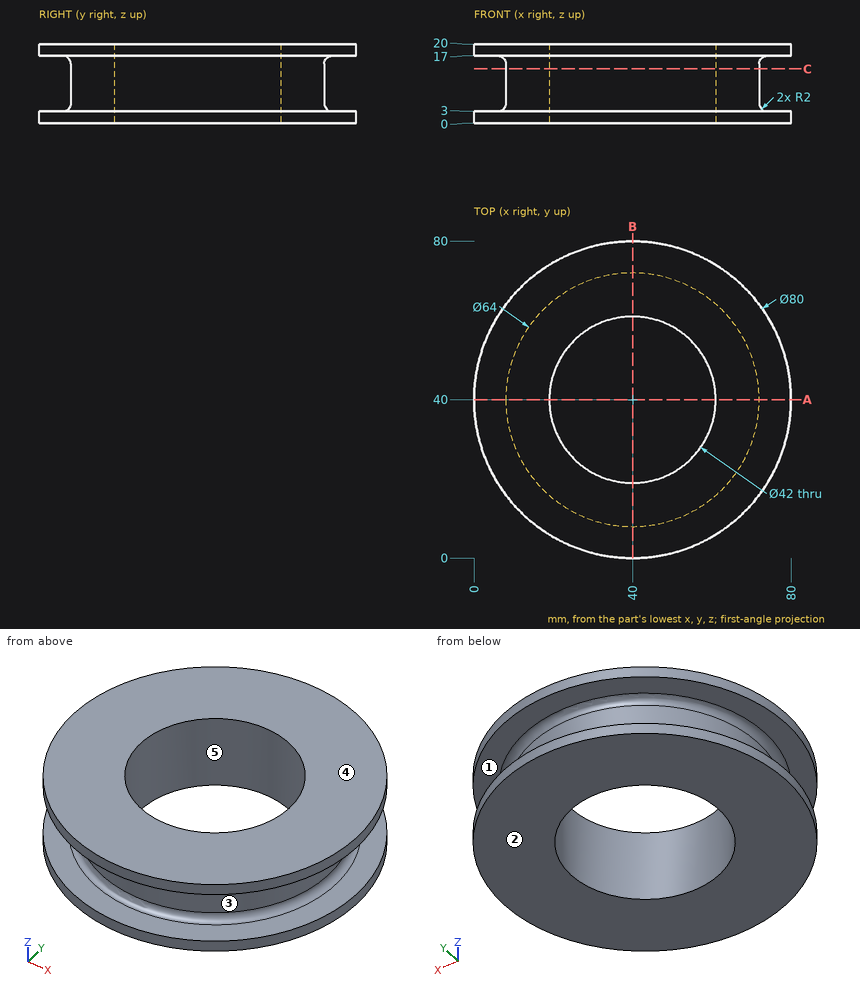
Study the drawing (mm; zero at the part's minimum x, y, z) and answer. A direction names the side the tool comes from. Give positions to 0.01 mm unless a question says otherwise; leave off trailing zeros. Loops run counter-clockwise (first coordinate to the right, second up) from the corner with the lowest first, then second, coordinate; pieces in that order, holes last. Notation, with made-up numbers: (76.5, 56) - (80.5, 56) arc R36 cw to (80.5, 92) - close; hole circle Ø10 at (-1, 61.25). An arc over 180 degrees is marked (long way). Answer in a Markdown table with one row per item. Add a question column.
Q1. Each of these flat-tipped pins is pushed along its axis until it touches: P1, Ø2, axis at y = 15.5, z = 2.5, coming from the +X side; P2, Ø5, axis at x = 24, z = 9.5, coming from the +Y side; P3, Ø1.5, axis at x = 35.5, y = 20.5, coming from the -Z side; P4, Ø3, axis at x = 19.5, z = 11, coming from the +Y side. Where does it stop, or does it pass through?
Q2. The part is cut by section C-C (z = 13.75). Determine the outline of the cut face in (x, y), and give its area (3 significant figures).
Q3. A tool of negligible diameter and unlimited length cuts with its end or side. For the marked faces 1 and 2, from which of +Z, -Z, +X, -X, +Y, -Y can it reach the whole face along a straight path? Write none if from no direction.
Q4. Consider line 1 along Y through (x, z) = (40, 10.75); line 2 along Y through (x, z) = (40, 4.5); line 3 along X through (y, z) = (21, 6.5). Determine where each line is inside the solid, lowest interval first.
Q5. Determine the mould class of the marked faces 3, 4 and 5 for opening direction X: released by +X, released by -X, zero draft, split by the parting line, or undercut.
Q6. The part is cut by section A-A (y = 40). Determine the outline of the cut face in (x, z), and give its area (3 significant figures).
Solution:
| question | item | result |
|---|---|---|
| 1 | P1 | stops at x = 72.37 |
| 1 | P2 | stops at y = 69.01 |
| 1 | P3 | passes through |
| 1 | P4 | stops at y = 65.75 |
| 2 | outline | circle Ø64 at (40, 40); hole circle Ø42 at (40, 40) |
| 2 | area | 1,830 mm² |
| 3 | face 1 | none |
| 3 | face 2 | -Z, +X, -X, +Y, -Y |
| 4 | line 1 | y = 8 to 19, 61 to 72 |
| 4 | line 2 | y = 7.94 to 19, 61 to 72.06 |
| 4 | line 3 | x = 14.25 to 31.06, 48.94 to 65.75 |
| 5 | face 3 | split by the parting line |
| 5 | face 4 | zero draft |
| 5 | face 5 | undercut |
| 6 | outline | (0, 0) - (19, 0) - (19, 20) - (0, 20) - (0, 17) - (6, 17) arc R2 cw to (8, 15) - (8, 5) arc R2 cw to (6, 3) - (0, 3) - close; (61, 0) - (80, 0) - (80, 3) - (74, 3) arc R2 cw to (72, 5) - (72, 15) arc R2 cw to (74, 17) - (80, 17) - (80, 20) - (61, 20) - close |
| 6 | area | 539 mm² |
